Input: dimensioned drawing with shaded views. Units: mm. Origin: part minimum x, y, z. A direction names the side the tool comes from. Round coordinates to 2 decimals unless told otherwise and drop trailing zeros. Order: outer loops, then holes, each group sorted by start corner. A loop starts at its lowest first (then second) coordinate and runs counter-clockwise, first axis right, second up. Notation, with made-up numbers: (59, -23.5) - (67, -23.5) arc R14 ccw to (67, -4.5) - close; hole circle Ø6 at (46, 36). An arc over 180 degrees is marked (long way). One line per item, written item: value. Start each with the question number.
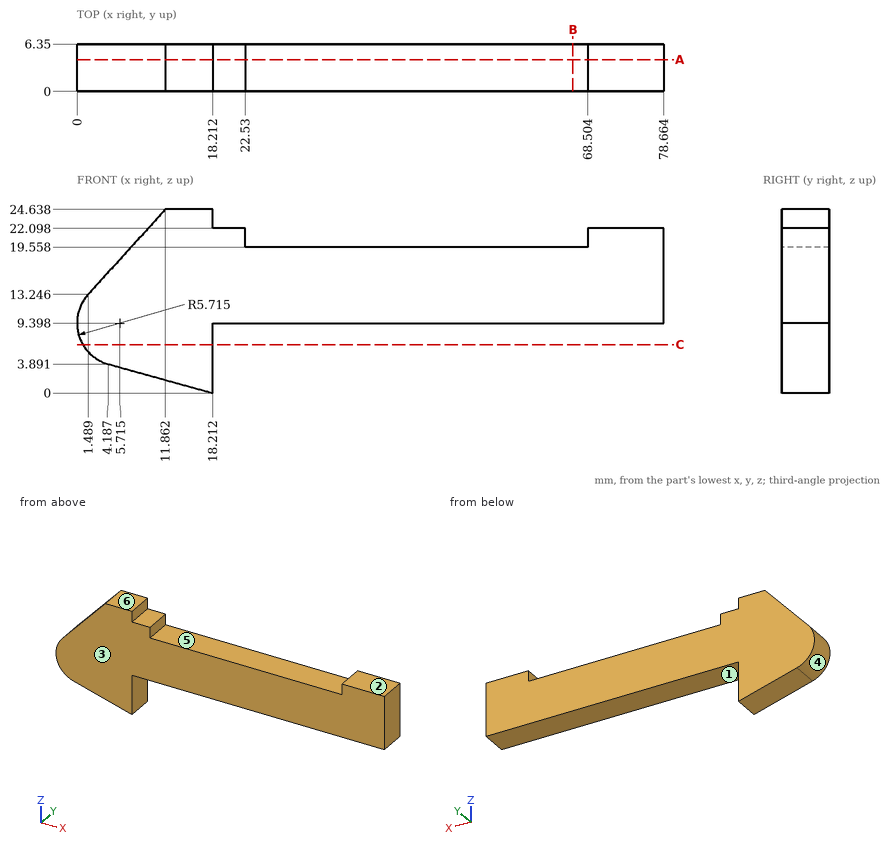
1. Set-up query: the marked faces 1, 2 and 3. Return all of +Z, -Z, +X, -X, +Y, -Y with unobstructed straight access to the full face (end or side cutting, diameter ignored); none if empty.
2. Pin query (flat end, axial travel): pin 1 (2 mm diameter, centred on y = 4.5, z = 23.5, fed in from +X); pin 2 (1.3 mm diameter, centred on y = 3.5, z = 21, fed in from -X); pin 3 (2 mm diameter, centred on x = 51, y = 2, fed in from -Z). Return the tip coordinate at first contact, or that it passes through.
3. Line query: line 1 (Z direction, x = 28.5, y = 2.75); line 2 (X direction, y = 4, z = 13.25) (1 decimal); line 3 (Z direction, x = 20, y = 4.5). Output: solid intervals per line, ascending. Write a range as from..to.
4. Section A-A (y = 4.25). Return the cut outline in (x, z) (1 decimal).
5. Section B-B (x = 66.5). Return the cut outline in (y, z).
6. Section C-C (z = 6.5). Return the cut outline in (x, y), then the cut area to 3 significant figures.
7. Pull-direction query (X, two-part tool) for the marked faces 4, 5 and 6; classes: released by +X, released by -X, zero draft, split by the parting line, or undercut.
Solved:
1. face 1: -Z, +X, +Y, -Y
1. face 2: +Z, +X, +Y, -Y
1. face 3: +Z, -Z, +X, -X, -Y
2. pin 1: stops at x = 18.21
2. pin 2: stops at x = 7.96
2. pin 3: stops at z = 9.4
3. line 1: z = 9.4..19.56
3. line 2: x = 1.5..78.7
3. line 3: z = 9.4..22.1
4. outline: (1.5, 13.2) arc R5.7 ccw to (4.2, 3.9) - (18.2, 0) - (18.2, 9.4) - (78.7, 9.4) - (78.7, 22.1) - (68.5, 22.1) - (68.5, 19.6) - (22.5, 19.6) - (22.5, 22.1) - (18.2, 22.1) - (18.2, 24.6) - (11.9, 24.6) - close
5. outline: (0, 9.4) - (6.35, 9.4) - (6.35, 19.56) - (0, 19.56) - close
6. outline: (0.79, 0) - (18.21, 0) - (18.21, 6.35) - (0.79, 6.35) - close
6. area: 111 mm²
7. face 4: released by -X
7. face 5: undercut
7. face 6: zero draft
